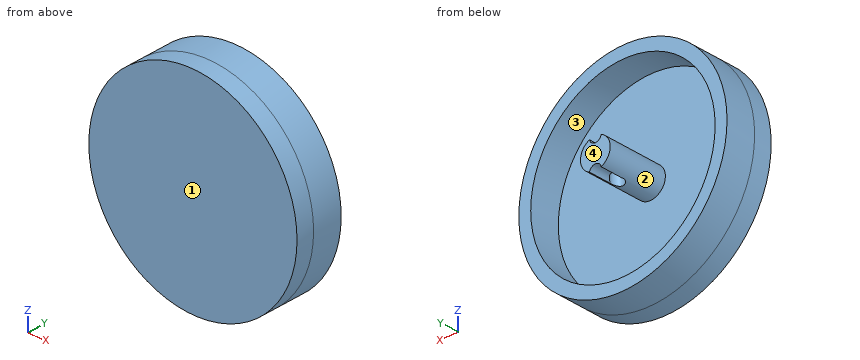
Autodesk Inventor part; units mm, degrees
ref_plane "YZ Plane" through (0, 0, 0) normal (1, 0, 0) x (0, 1, 0)
ref_plane "XZ Plane" through (0, 0, 0) normal (0, 1, 0) x (-1, 0, 0)
ref_plane "XY Plane" through (0, 0, 0) normal (0, 0, 1) x (1, 0, 0)
sketch "Sketch1" plane through (0, 0, 0) normal (0, 1, 0) x (-1, 0, 0)
  circle A0 centre (0, 0) radius 17.5
  dimension "d0" = 35
extrude "Extrusion1" add sketch "Sketch1" along normal blind 3
sketch "Sketch2" plane through (0, 3, 0) normal (0, 1, 0) x (1, 0, 0)
  circle A0 centre (0, 0) radius 17.5
  circle A1 centre (0, 0) radius 2.5
  dimension "d3" = 5
extrude "Extrusion2" add sketch "Sketch2" along normal blind 10 contours A1
sketch "Sketch3" plane through (0, 0, 0) normal (0, 0, 1) x (1, 0, 0)
  circle A0 centre (0, 9) radius 1
  line L0 (2.5, 13) -> (-2.5, 13)
  point P0 (0, 0)
  dimension "d6" = 2
  dimension "d9" = 4
extrude "Extrusion3" cut sketch "Sketch3" along normal through all both and the other way through all
sketch "Sketch4" plane through (0, 13, 0) normal (0, 1, 0) x (1, 0, 0)
  circle A0 centre (0, 0) radius 2.5
  circle A1 centre (0, 2.5) radius 1
  circle A2 centre (0, -2.5) radius 1
  dimension "d10" = 2
extrude "Extrusion4" cut sketch "Sketch4" against normal blind 4 contours A1 A0 | A0 A1 | A2 A0 | A0 A2
sketch "Sketch5" plane through (0, 3, 0) normal (0, 1, 0) x (1, 0, 0)
  circle A0 centre (0, 0) radius 17.5
  circle A1 centre (0, 0) radius 15.5
  dimension "d13" = 2
extrude "Extrusion5" add sketch "Sketch5" along normal blind 5
properties part number "pot_bottom"
Geometry check sheet. Reference: the model listing, model coordinates, mm. Face numbers are marked on the shaded views. A direction names the side the tool comes from. Give positions to 0.01 mm unless a question says otherwise; leave off trailing zeros. Loops run counter-clockwise (first coordinate to the right, second up) from the corner with the lowest first, then second, coordinate; pieces in that order, holes last. Notation, with made-up numbers: (-20, 28) -> (18, 28) arc R16 ccw to (18, 53) -> close; hole circle Ø10 at (11, 47.25). An arc over 180 degrees is marked (long way). Answer in a Markdown table with one row per item. Add a question column.
1) Set-up check for the marked faces 1 and 2: record each of +Z, -Z, +X, -X, +Y, -Y from which the full face is reachable in a straight line by a thin tool's end or side.
2) Material ranges on probe 1 along Z at (x, y) = (0, 5.4); probe 2 along Y at (x, z) = (0, 1.25); probe 3 along X at (y, z) = (6.5, -2), recorded low to high. Write a range as from..to.
3) Cross-section at D-D on z = 11.5. Record the boundary of the cut face in (x, y).
4) Draft check along X on the marked faces 3 and 4. Enter one of: pulls with the +X half, pulls with the -X half, needs draft (parallel to the pull), parting line crosses it, or undercut.
5) Cross-section at B-B on y = 5.75. Record the boundary of the cut face in (x, z), and give its area (3 significant figures).
6) Cross-section at C-C on x = 0. Record the boundary of the cut face in (y, z).
7) Cross-section at A-A on z = 0. Record the boundary of the cut face in (x, y).
8) Gauge pin test, flat ends, axial feed: P1, Ø1.5, axis at y = 5, z = -0.5, coming from the +X side; P2, Ø5, axis at y = 4, z = 7, coming from the +X side; P3, Ø12, axis at x = -13, z = -5, coming from the +Y side; P4, Ø6, axis at x = 9, y = 10.5, coming from the +Z side. Record the tip position at first contact, or that the pin passes through.
Outcome:
| question | item | result |
|---|---|---|
| 1 | face 1 | +Z, -Z, +X, -X, -Y |
| 1 | face 2 | +Y |
| 2 | probe 1 | z = -17.5..-15.5, -2.5..2.5, 15.5..17.5 |
| 2 | probe 2 | y = 0..8, 10..13 |
| 2 | probe 3 | x = -17.39..-15.37, -1.5..1.5, 15.37..17.39 |
| 3 | outline | (-13.19, 0) -> (13.19, 0) -> (13.19, 8) -> (10.39, 8) -> (10.39, 3) -> (-10.39, 3) -> (-10.39, 8) -> (-13.19, 8) -> close |
| 4 | face 3 | undercut |
| 4 | face 4 | needs draft |
| 5 | outline | circle Ø35 at (0, 0); circle Ø5 at (0, 0); hole circle Ø31 at (0, 0) |
| 5 | area | 227 mm^2 |
| 6 | outline | (0, -17.5) -> (8, -17.5) -> (8, -15.5) -> (3, -15.5) -> (3, -2.5) -> (8, -2.5) -> (8, 2.5) -> (3, 2.5) -> (3, 15.5) -> (8, 15.5) -> (8, 17.5) -> (0, 17.5) -> close; (10, -1.5) -> (13, -1.5) -> (13, 1.5) -> (10, 1.5) -> close |
| 7 | outline | (-17.5, 0) -> (17.5, 0) -> (17.5, 8) -> (15.5, 8) -> (15.5, 3) -> (2.5, 3) -> (2.5, 13) -> (-2.5, 13) -> (-2.5, 3) -> (-15.5, 3) -> (-15.5, 8) -> (-17.5, 8) -> close; hole circle Ø2 at (0, 9) |
| 8 | P1 | stops at x = 17.5 |
| 8 | P2 | stops at x = 16.91 |
| 8 | P3 | stops at y = 8 |
| 8 | P4 | stops at z = 15.89 |
